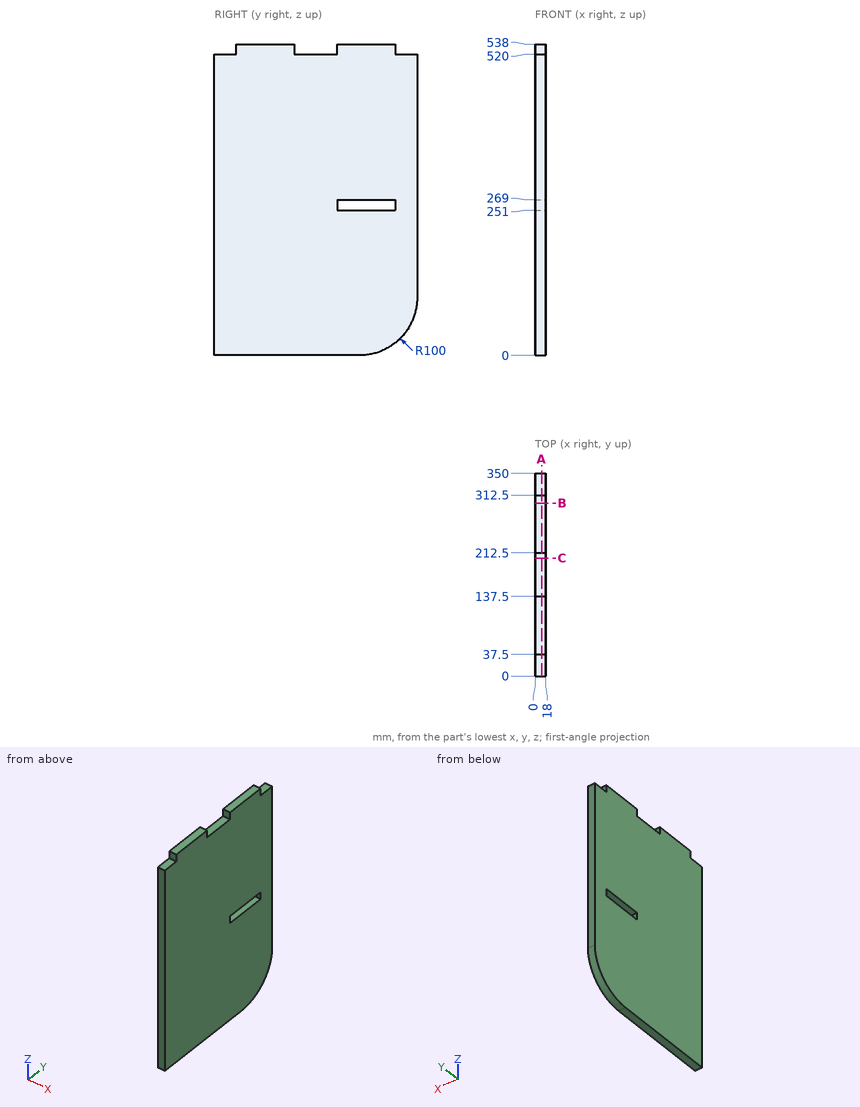
The figure shows three views and two pictorial views of one solid part (mm, origin at its lowest corner). Answer the questions. Round coordinates to 2 decimals unless told otherwise and drop trailing zeros. Order: outer loops, then holes, each group sorted by start corner. A loop starts at its lowest first (then second) coordinate and runs counter-clockwise, first axis right, second up.
Q1. Given pin 1 Ø9 at (x, z) = (10.5, 525) entering from -Y; pin 2 Ø3 at (x, y) = (15, 269.5) entering from -Z; pin 3 Ø5.5 at (x, y) = (6.5, 285.5) entering from -Z, each flat-ended and moving along its own axis, determine where each tip first touches the part or whether it passes through.
Solution:
pin 1: stops at y = 37.5
pin 2: stops at z = 1.63
pin 3: stops at z = 5.51
Q2. Find the intervals of material crossed by line 1 along Y through (x, z) = (6.5, 268.5); line 2 along Z through (x, y) = (2.75, 153); line 3 along Z through (x, y) = (10.5, 262.5), in increasing order.
Solution:
line 1: y = 0 to 212.5, 312.5 to 350
line 2: z = 0 to 520
line 3: z = 0.78 to 251, 269 to 538
Q3. A cutting plane is placed at B-B, the plane y = 298.5. Determine the outline of the cut face in (x, z).
Solution:
outline: (0, 12.55) - (18, 12.55) - (18, 251) - (0, 251) - close; (0, 269) - (18, 269) - (18, 538) - (0, 538) - close
Q4. A cutting plane is placed at A-A, the plane x = 11.5. Determine the outline of the cut face in (y, z).
Solution:
outline: (0, 0) - (250, 0) arc R100 ccw to (350, 100) - (350, 520) - (312.5, 520) - (312.5, 538) - (212.5, 538) - (212.5, 520) - (137.5, 520) - (137.5, 538) - (37.5, 538) - (37.5, 520) - (0, 520) - close; hole (212.5, 251) - (312.5, 251) - (312.5, 269) - (212.5, 269) - close
Q5. A cutting plane is placed at C-C, the plane y = 203.5. Determine the outline of the cut face in (x, z), then the cut area to 3 significant figures.
Solution:
outline: (0, 0) - (18, 0) - (18, 520) - (0, 520) - close
area: 9,360 mm2
